```python
from build123d import *

# Parameters (mm, degrees)
BOSS_EXTRUDE1_DEPTH = 254
SKETCH2_R           = 4.365625
CUT_EXTRUDE1_DEPTH  = 3.175
SKETCH3_R           = 4.365625
CUT_EXTRUDE2_DEPTH  = 3.175


with BuildPart() as part:
    # Sketch1 → Boss-Extrude1 (new body)
    with BuildSketch(Plane(origin=(0, 0, 0), x_dir=(0, 0, -1), z_dir=(1, 0, 0))):
        Polygon((-3.175, 0), (-50.8, 0), (-50.8, -3.175), (0, -3.175), (0, 0), (0, 47.625), (-3.175, 47.625), align=None)
    extrude(amount=BOSS_EXTRUDE1_DEPTH)

    # Sketch2 → Cut-Extrude1 (cut)
    with BuildSketch(Plane.XY.offset(3.175)):
        with Locations((177.8, 23.8125)):
            Circle(SKETCH2_R)
        with Locations((215.9, 23.8125)):
            Circle(SKETCH2_R)
    extrude(amount=-CUT_EXTRUDE1_DEPTH, mode=Mode.SUBTRACT)

    # Sketch3 → Cut-Extrude2 (cut)
    with BuildSketch(Plane(origin=(0, 0, 0), x_dir=(1, 0, 0), z_dir=(0, 1, 0))):
        with Locations((177.8, -26.9875)):
            Circle(SKETCH3_R)
        with Locations((215.9, -26.9875)):
            Circle(SKETCH3_R)
    extrude(amount=-CUT_EXTRUDE2_DEPTH, mode=Mode.SUBTRACT)


solid = part.part
```
Work out the finished part from the listing and answer in its coordinate system (mm). A direction names the side the tool comes from. Give positions to 0.01 mm unless a question says otherwise; leave off trailing zeros. Loops run counter-clockwise (first coordinate to the right, second up) from the corner with the lowest first, then second, coordinate; pieces in that order, holes last. Notation, with made-up numbers: (-14, 46.25) -> (-9, 46.25) arc R26 ccw to (-9, 66.25) -> close; hole circle Ø2 at (15.25, 11.25). An arc over 180 degrees is marked (long way). Put each result on its own line as item: value. Start each with the question number.
Item 1: The part is cut by section A-A (x = 177.8). Give the vertices of the cut face in (y, z) (3 decimals), then the cut area to 3 significant figures.
Item 2: The part is cut by section C-C (z = 47.5). Give the vertices of the cut face in (x, y) (3 decimals), then the cut area to 3 significant figures.
Item 3: Each of these flat-tipped pins is pushed along its axis until it touches: P1, Ø10, axis at x = 177.8, z = 26.99, coming from the +Y side; P2, Ø2, axis at x = 126.5, y = 29.5, coming from the +Z side (3 decimals). Where does it stop, or does it pass through?
Item 4: The mould has two halves that part along Z. Classify faces 3 (the face through (219.933, 22.14, 1.61)), 4 (the face through (125, 24, 3.175)), 5 (the face through (173.44, -1.57, 26.8)): released by +Z, released by -Z, zero draft, split by the parting line, or undercut.
Item 5: Which of the six approach directions +Z, -Z, +X, -X, +Y, -Y give full straight-line access (tool end or side, diameter ignored) to faces 1 (the face through (125, -3.175, 26)), 2 (the face through (125, 0, 27))?
Item 6: The part is cut by section B-B (x = 232). Give the vertices of the cut face in (y, z) (3 decimals), then the cut area to 4 significant figures.
Item 7: The part is cut by section D-D (y = 43). Give the vertices of the cut face in (x, z) (3 decimals).
Item 8: Find the intervals of material crossed by L1, parallel to Y at x = 177.8, z = 2.25 (3 decimals); L2, parallel to Z at x = 177.8, y = -0.9; L3, parallel to Z at x = 117, y = 37.5 (3 decimals), in increasing order. Write a range as [from, to].
Answers below:
1. outline: (-3.175, 0) -> (19.447, 0) -> (19.447, 3.175) -> (0, 3.175) -> (0, 22.622) -> (-3.175, 22.622) -> close; (-3.175, 31.353) -> (0, 31.353) -> (0, 50.8) -> (-3.175, 50.8) -> close; (28.178, 0) -> (47.625, 0) -> (47.625, 3.175) -> (28.178, 3.175) -> close
1. area: 257 mm2
2. outline: (0, -3.175) -> (254, -3.175) -> (254, 0) -> (0, 0) -> close
2. area: 806 mm2
3. P1: y = 0
3. P2: z = 3.175
4. face 3: zero draft
4. face 4: released by +Z
4. face 5: undercut
5. face 1: +Z, -Z, +X, -X, -Y
5. face 2: +Z, +X, -X, +Y
6. outline: (-3.175, 0) -> (47.625, 0) -> (47.625, 3.175) -> (0, 3.175) -> (0, 50.8) -> (-3.175, 50.8) -> close
6. area: 312.5 mm2
7. outline: (0, 0) -> (254, 0) -> (254, 3.175) -> (0, 3.175) -> close
8. L1: [-3.175, 19.447], [28.178, 47.625]
8. L2: [0, 22.62], [31.35, 50.8]
8. L3: [0, 3.175]
